Design review of the part built by this model. Coordinates are the model's own, in mm. A direction names the side the tool comes from. Coordinates: 2 decimals unless noted, no trailing zeros. Write each loop counter-clockwise with the first axis right and the second up, starting at its lowest first coordinate (ties: lowest second). Pieces come first, ordered by that corner, then holes.
Q1. Clearance check with flat-ended pins moving along their axes: pin 1 Ø1.5 at (y, z) = (2, -4) entering from -X; pin 2 Ø9.5 at (x, y) = (-26, 5) entering from -Z; pin 3 Ø3 at (x, z) = (-18, -6.5) entering from -Y; pin 4 Ø8 at (x, y) = (-33, 12) entering from +Z. State where each tip first meets the part, or that it passes through.
Q2. Add section A-A, the plane x = -32. Give the boundary of the cut face in (y, z).
Q3. Add section B-B, the plane x = -11. Give the boundary of the cut face in (y, z), plus the area to 3 significant figures.
Q4. Add section D-D, the plane z = 1. Give the boundary of the cut face in (x, y).
Q5. To check wall thickness, follow probe 1 along Z at (x, y) = (-24, -0.5); probe 2 along Z at (x, y) = (-17, 14); probe 3 along Y at (x, z) = (-22, 7.25). State the ranges of each line that lie inside material, in increasing order.
Q6. Machinability: for faces 1 (the face through (-21.962, 3.887, -4.93)), 2 (the face through (-21.542, 11.352, 7.395)), 3 (the face through (-6.752, 6, 3)), which of the approach directions +Z, -Z, +X, -X, +Y, -Y give a long, thin tool a straight path to every point of the face, cutting with its end or side? Answer none if there is none.
Q7. Add section C-C, the plane y = 1.25. Give the boundary of the cut face in (x, z).
from build123d import *

# Parameters (mm, degrees)
BOSS_EXTRUDE1_DEPTH = 15
BOSS_EXTRUDE2_DEPTH = 10


with BuildPart() as part:
    # Sketch1 → Boss-Extrude1 (new body)
    with BuildSketch(Plane.XY):
        Polygon((-36.752136752, 6.282051282), (-36.752136752, -3.717948718), (-6.752136752, -3.717948718), (-6.752136752, 16.282051282), align=None)
    extrude(amount=BOSS_EXTRUDE1_DEPTH)

    # Sketch2 → Boss-Extrude2 (add)
    with BuildSketch(Plane(origin=(0, 0, 0), x_dir=(-1, 0, 0), z_dir=(0, 0, -1))):
        Polygon((6.752136752, -3.717948718), (6.752136752, 16.282051282), (36.752136752, 16.282051282), (36.752136752, 11.282051282), align=None)
    extrude(amount=BOSS_EXTRUDE2_DEPTH)


solid = part.part
Here are the results:
1. pin 1: stops at x = -19.69
1. pin 2: stops at z = -10
1. pin 3: stops at y = 1.16
1. pin 4: stops at z = 0
2. outline: (-3.72, 0) - (7.87, 0) - (7.87, 15) - (-3.72, 15) - close; (8.91, -10) - (16.28, -10) - (16.28, 0) - (8.91, 0) - close
3. outline: (-3.72, 0) - (-1.59, 0) - (-1.59, -10) - (16.28, -10) - (16.28, 0) - (14.87, 0) - (14.87, 15) - (-3.72, 15) - close
3. area: 458 mm2
4. outline: (-36.75, -3.72) - (-6.75, -3.72) - (-6.75, 16.28) - (-36.75, 6.28) - close
5. probe 1: z = 0 to 15
5. probe 2: z = -10 to 0
5. probe 3: y = -3.72 to 11.2
6. face 1: -Z, -X, -Y
6. face 2: +Z, -X, +Y
6. face 3: +Z, -Z, +X, +Y, -Y
7. outline: (-36.75, 0) - (-16.69, 0) - (-16.69, -10) - (-6.75, -10) - (-6.75, 15) - (-36.75, 15) - close
